The model under review builds one solid part; all positions refer to its coordinate system, in mm. A direction names the side the tool comes from. Round coordinates to 2 decimals unless told otherwise and drop trailing zeros. Loops run counter-clockwise (first coordinate to the right, second up) from the corner with the lowest first, then second, coordinate; pieces in that order, holes last. Notation, with made-up numbers: (-19, -28) -> (35, -28) arc R19 cw to (35, -4) -> close; hole circle Ø1 at (-38, -12.5). An arc over 180 degrees is marked (long way). Write each question's results on one line, items separated by ' | '. Start each with the question number.
Item 1: Clearance check with flat-ended pins moving along their axes: pin 1 Ø10 at (x, y) = (-194.5, 11) entering from +Z; pin 2 Ø8 at (x, y) = (-292.5, 5.5) entering from -Z; pin 3 Ø8 at (x, z) = (-174.5, 46.5) entering from -Y; pin 4 Ø3 at (x, y) = (-232.09, 9.52) entering from +Z. State where each tip first meets the part, or that it passes through.
Item 2: For L1, parallel to Z at x = -150.5, y = 7.75; L2, parallel to X at y = 4, z = 161.5; L3, parallel to X at y = 17.75, z = 129, list the stretches that pass through material, from the lowest coordinate up. Write a range as from..to.
Item 3: Mouldability with a two-part tool opening along Z and no side actions: class faces 1 (the flat face through (-140.828, 16, 130)), 2 (the flat face through (-245.87, 9.39, 248.57)), 3 (the flat face through (-281.964, 6, 129)) as pulls with the +Z half, pulls with the -Z half, needs draft (parallel to the pull), parting line crosses it, or undercut.
Item 4: We need section A-A (z = 76). Give the boundary of the cut face in (x, y), and give its area (3 significant figures).
Item 5: We need section B-B (x = -178). Give the boundary of the cut face in (y, z).
Item 6: We need section C-C (x = -270). Give the boundary of the cut face in (y, z), and give its area (3 significant figures).
Item 7: We need section D-D (z = 20). Give the boundary of the cut face in (x, y) (3 decimals).
Item 8: Tool access review of faces 4 (the flat face through (-306.818, 9, 164)), 5 (the flat face through (-289.584, -4, 128)), 6 (the cylindrical face through (-311.827, 11.051, 167.706)): name each direction out of +Z, -Z, +X, -X, +Y, -Y from which nothing blocks a thin tool from reaching the whole face with its end or side.
from build123d import *

# Parameters (mm, degrees)
BOSS_EXTRUDE1_DEPTH     = 19.05
SKETCH2_R               = 1.7526
CUT_EXTRUDE1_DEPTH      = 221.7
SKETCH3_R               = 5.08
CUT_EXTRUDE2_DEPTH      = 170.7
CIRPATTERN1_START       = -323.388650449
CIRPATTERN1_OUTLINE_R   = 5.08
CIRPATTERN1_DEPTH       = 29.913478247
CIRPATTERN1_START_2     = -293.475172202
CIRPATTERN1_2_OUTLINE_R = 1.7526
CIRPATTERN1_2_DEPTH     = 11.511586101
SKETCH5_R               = 1.7526
CUT_EXTRUDE3_DEPTH      = 295.91
SKETCH6_R               = 1.7526
CUT_EXTRUDE4_DEPTH      = 20.574
SKETCH7_R               = 5.08
CUT_EXTRUDE5_DEPTH      = 10.16
CIRPATTERN2_COUNT       = 2
SKETCH8_W               = 6.182053834
SKETCH8_H               = 6.581850062
SKETCH8_R               = 1.7526
BOSS_EXTRUDE2_DEPTH     = 7.62
CIRPATTERN3_COUNT       = 2


# Read off the part's stored shape, not the designer's step: CirPattern1
with BuildPart() as part:
    # Sketch1 → Boss-Extrude1 (new body)
    with BuildSketch(Plane(origin=(0, 0, 0), x_dir=(1, 0, 0), z_dir=(0, 1, 0))):
        with BuildLine():
            Line((-238.437586101, -1.254416157), (-253.074790503, -15.891620559))
            ThreePointArc((-253.074790503, -15.891620559), (-292.273480014, -31.022056532), (-323.388650449, -59.258797155))
            Line((-323.388650449, -59.258797155), (-323.388650449, -198.000222119))
            ThreePointArc((-323.388650449, -198.000222119), (-292.280058459, -226.218805317), (-253.09778688, -241.344364055))
            Line((-253.09778688, -241.344364055), (-253.074790503, -241.367360432))
            Line((-253.074790503, -241.367360432), (-238.437586101, -256.004564834))
            Line((-238.437586101, -256.004564834), (-225.737586101, -256.004564834))
            Line((-225.737586101, -256.004564834), (-211.100381699, -241.367360432))
            Line((-211.100381699, -241.367360432), (-211.077385322, -241.344364055))
            ThreePointArc((-211.077385322, -241.344364055), (-171.924255518, -226.236769292), (-140.827968899, -198.054719126))
            Line((-140.827968899, -198.054719126), (-140.827968899, -59.204261865))
            ThreePointArc((-140.827968899, -59.204261865), (-171.930845296, -31.004081905), (-211.100381699, -15.891620559))
            Line((-211.100381699, -15.891620559), (-225.737586101, -1.254416157))
            Line((-225.737586101, -1.254416157), (-238.437586101, -1.254416157))
        make_face()
        with BuildLine():
            Line((-281.963586101, -124.819490495), (-306.818249022, -115.773133009))
            Line((-306.818249022, -115.773133009), (-306.818249022, -59.258790155))
            ThreePointArc((-306.818249022, -59.258790155), (-232.087586101, -26.656188726), (-157.356923179, -59.258790155))
            Line((-157.356923179, -59.258790155), (-157.356923179, -115.773133009))
            Line((-157.356923179, -115.773133009), (-182.211586101, -124.819490495))
            Line((-182.211586101, -124.819490495), (-182.211586101, -132.439490495))
            Line((-182.211586101, -132.439490495), (-157.356923179, -141.485847982))
            Line((-157.356923179, -141.485847982), (-157.356923179, -198.054719126))
            ThreePointArc((-157.356923179, -198.054719126), (-232.087586101, -230.624332183), (-306.818249022, -198.054719126))
            Line((-306.818249022, -198.054719126), (-306.818249022, -141.485847982))
            Line((-306.818249022, -141.485847982), (-281.963586101, -132.439490495))
            Line((-281.963586101, -132.439490495), (-281.963586101, -124.819490495))
        make_face(mode=Mode.SUBTRACT)
    extrude(amount=BOSS_EXTRUDE1_DEPTH)

    # Sketch2 → Cut-Extrude1 (cut)
    with BuildSketch(Plane(origin=(0, 0, 0), x_dir=(0, 0, -1), z_dir=(1, 0, 0))):
        with Locations((-128.653847867, 9.576501184)):
            Circle(SKETCH2_R)
    extrude(amount=-CUT_EXTRUDE1_DEPTH, mode=Mode.SUBTRACT)

    # Sketch3 → Cut-Extrude2 (cut)
    with BuildSketch(Plane(origin=(0, 0, 0), x_dir=(0, 0, -1), z_dir=(1, 0, 0))):
        with Locations((-128.653847867, 9.576501184)):
            Circle(SKETCH3_R)
    extrude(amount=-CUT_EXTRUDE2_DEPTH, mode=Mode.SUBTRACT)

    # CirPattern1 outline → CirPattern1 (cut)
    with BuildSketch(Plane.YZ.offset(CIRPATTERN1_START)):
        with Locations((9.576501184, 128.605133124)):
            Circle(CIRPATTERN1_OUTLINE_R)
    extrude(amount=CIRPATTERN1_DEPTH, mode=Mode.SUBTRACT)

    # CirPattern1 2 outline → CirPattern1 2 (cut)
    with BuildSketch(Plane.YZ.offset(CIRPATTERN1_START_2)):
        with Locations((9.576501184, 128.605133124)):
            Circle(CIRPATTERN1_2_OUTLINE_R)
    extrude(amount=CIRPATTERN1_2_DEPTH, mode=Mode.SUBTRACT)

    # Sketch5 → Cut-Extrude3 (cut)
    with BuildSketch(Plane(origin=(0, 0, 1.254416157), x_dir=(-1, 0, 0), z_dir=(0, 0, -1))):
        with Locations((232.087586101, 9.525)):
            Circle(SKETCH5_R)
    extrude(amount=-CUT_EXTRUDE3_DEPTH, mode=Mode.SUBTRACT)

    # Sketch6 → Cut-Extrude4 (cut)
    with BuildSketch(Plane.ZY.offset(157.356923179)):
        with Locations((84.658797155, 9.525)):
            Circle(SKETCH6_R)
    cut_extrude4 = extrude(amount=-CUT_EXTRUDE4_DEPTH, mode=Mode.SUBTRACT)

    # Sketch7 → Cut-Extrude5 (cut)
    with BuildSketch(Plane.ZY.offset(157.356923179)):
        with Locations((84.658797155, 9.525)):
            Circle(SKETCH7_R)
    cut_extrude5 = extrude(amount=-CUT_EXTRUDE5_DEPTH, mode=Mode.SUBTRACT)

    # CirPattern2: Cut-Extrude4, Cut-Extrude5 ×2 about axis
    cirpattern2_axis = Axis((-232.087586101, 0, 128.605133124), (0, -1, 0))
    add([cut_extrude4.rotate(cirpattern2_axis, i * 360 / CIRPATTERN2_COUNT) for i in range(1, CIRPATTERN2_COUNT)], mode=Mode.SUBTRACT)
    add([cut_extrude5.rotate(cirpattern2_axis, i * 360 / CIRPATTERN2_COUNT) for i in range(1, CIRPATTERN2_COUNT)], mode=Mode.SUBTRACT)

    # Sketch8 → Boss-Extrude2 (add)
    with BuildSketch(Plane(origin=(-281.963586101, 0, 0), x_dir=(0, 0, -1), z_dir=(1, 0, 0))):
        with Locations((-129.348463578, -3.290925031)):
            Rectangle(SKETCH8_W, SKETCH8_H)
        with Locations((-129.752447072, -3.098573281)):
            Circle(SKETCH8_R, mode=Mode.SUBTRACT)
    boss_extrude2 = extrude(amount=-BOSS_EXTRUDE2_DEPTH)

    # CirPattern3: Boss-Extrude2 ×2 about axis
    cirpattern3_axis = Axis((-232.087586101, 0, 128.605133124), (0, 1, 0))
    for i in range(1, CIRPATTERN3_COUNT):
        add(boss_extrude2.rotate(cirpattern3_axis, i * 360 / CIRPATTERN3_COUNT))


solid = part.part
Here are the results:
1) pin 1: stops at z = 238.56 | pin 2: stops at z = 28.79 | pin 3: stops at y = 0 | pin 4: passes through
2) L1: z = 48.06..79.9, 89.42..123.91, 133.39..209.2 | L2: x = -323.39..-306.82, -157.36..-140.83 | L3: x = -323.39..-281.96, -182.21..-140.83
3) face 1: needs draft | face 2: pulls with the +Z half | face 3: undercut
4) outline: (-323.39, 0) -> (-306.82, 0) -> (-306.82, 19.05) -> (-323.39, 19.05) -> close; (-157.36, 0) -> (-140.83, 0) -> (-140.83, 19.05) -> (-157.36, 19.05) -> close | area: 631 mm2
5) outline: (-6.58, 124.77) -> (0, 124.77) -> (0, 123.29) -> (19.05, 123.29) -> (19.05, 133.97) -> (0, 133.97) -> (0, 130.95) -> (-6.58, 130.95) -> close; (0, 27.51) -> (19.05, 27.51) -> (19.05, 42.19) -> (0, 42.19) -> close; (0, 215.11) -> (19.05, 215.11) -> (19.05, 229.73) -> (0, 229.73) -> close; hole circle Ø3.51 at (-3.1, 127.46); hole circle Ø3.51 at (9.58, 128.65)
6) outline: (0, 20.4) -> (19.05, 20.4) -> (19.05, 33.97) -> (0, 33.97) -> close; (0, 223.32) -> (19.05, 223.32) -> (19.05, 236.84) -> (0, 236.84) -> close | area: 516 mm2
7) outline: (-268.826, 0) -> (-195.349, 0) -> (-195.349, 19.05) -> (-268.826, 19.05) -> close; hole circle Ø3.505 at (-232.088, 9.525)
8) face 4: +Y, -Y | face 5: +Z, -Z, -X, -Y | face 6: none
